Build history of the part. All positions in model axes, mm. Round coordinates to 2 decimals unless told otherwise and drop trailing zeros. Write each loop counter-clockwise with the first axis right and the second up, starting at its lowest first coordinate (ties: lowest second). Pieces come first, ordered by that corner, then holes. Notation, with made-up numbers: M -11.75,-36 L 14.25,-36 A11 ccw 14.25,-30 Z; hole C 70,-32.75 d5. An arc over 180 degrees is marked long. Write item = value, one per line.
Autodesk Inventor part; units mm, degrees
ref_plane "MP_XY" through (0, 0, 0) normal (0, 0, 1) x (1, 0, 0)
ref_plane "MP_YZ" through (0, 0, 0) normal (1, 0, 0) x (0, 1, 0)
ref_plane "MP_ZX" through (0, 0, 0) normal (0, 1, 0) x (0, 0, 1)
sketch "Sketch_12" plane through (0, 0, 0) normal (0, 0, 1) x (1, 0, 0)
  line L0 (-275, 538.5) -> (-275, 11.5)
  line L1 (-275, 11.5) -> (-273.5, 11.5)
  line L2 (-273.5, 11.5) -> (-263.9737, -5)
  line L3 (-263.9737, -5) -> (-255.5, -5)
  line L4 (-255.5, -5) -> (-255.5, 0)
  arc A0 (-244.5, 0) -> (-255.5, 0) centre (-250, 0) ccw
  line L5 (-244.5, 0) -> (-244.5, -12.5)
  line L6 (-244.5, -12.5) -> (244.5, -12.5)
  line L7 (244.5, -12.5) -> (244.5, 0)
  arc A1 (255.5, 0) -> (244.5, 0) centre (250, 0) ccw
  line L8 (255.5, 0) -> (255.5, -5)
  line L9 (255.5, -5) -> (263.9737, -5)
  line L10 (263.9737, -5) -> (273.5, 11.5)
  line L11 (273.5, 11.5) -> (275, 11.5)
  line L12 (275, 11.5) -> (275, 538.5)
  line L13 (275, 538.5) -> (273.5, 538.5)
  line L14 (273.5, 538.5) -> (263.9737, 555)
  line L15 (263.9737, 555) -> (255.5, 555)
  line L16 (255.5, 555) -> (255.5, 550)
  arc A2 (244.5, 550) -> (255.5, 550) centre (250, 550) ccw
  line L17 (244.5, 550) -> (244.5, 562.5)
  line L18 (244.5, 562.5) -> (-244.5, 562.5)
  line L19 (-244.5, 562.5) -> (-244.5, 550)
  arc A3 (-255.5, 550) -> (-244.5, 550) centre (-250, 550) ccw
  line L20 (-255.5, 550) -> (-255.5, 555)
  line L21 (-255.5, 555) -> (-263.9737, 555)
  line L22 (-263.9737, 555) -> (-273.5, 538.5)
  line L23 (-273.5, 538.5) -> (-275, 538.5)
  arc A4 (216.8088, 4.2) -> (216.8088, -4.2) centre (210, 0) ccw
  line L24 (216.8088, -4.2) -> (229, -4.2)
  line L25 (229, -4.2) -> (229, 4.2)
  line L26 (229, 4.2) -> (216.8088, 4.2)
  arc A5 (216.8088, 554.2) -> (216.8088, 545.8) centre (210, 550) ccw
  line L27 (216.8088, 545.8) -> (229, 545.8)
  line L28 (229, 545.8) -> (229, 554.2)
  line L29 (229, 554.2) -> (216.8088, 554.2)
  line L30 (-229, 4.2) -> (-229, -4.2)
  line L31 (-229, -4.2) -> (-216.8088, -4.2)
  arc A6 (-216.8088, -4.2) -> (-216.8088, 4.2) centre (-210, 0) ccw
  line L32 (-216.8088, 4.2) -> (-229, 4.2)
  line L33 (-229, 554.2) -> (-229, 545.8)
  line L34 (-229, 545.8) -> (-216.8088, 545.8)
  arc A7 (-216.8088, 545.8) -> (-216.8088, 554.2) centre (-210, 550) ccw
  line L35 (-216.8088, 554.2) -> (-229, 554.2)
extrude "Extrusion1" add sketch "Sketch_12" against normal blind 2.5
ref_plane "MP_XY" through (0, 0, 0) normal (0, 0, 1) x (1, 0, 0)
ref_plane "MP_YZ" through (0, 0, 0) normal (1, 0, 0) x (0, 1, 0)
ref_plane "MP_ZX" through (0, 0, 0) normal (0, 1, 0) x (0, 0, 1)
ref_plane "to_EB_XY" through (224.8, 0, -2.5) normal (0, 0, 1) x (1, 0, 0)
ref_plane "to_EB_YZ" through (224.8, 0, -2.5) normal (1, 0, 0) x (0, 1, 0)
ref_plane "to_EB_ZX" through (224.8, 0, -2.5) normal (0, 1, 0) x (0, 0, 1)
properties part number "166X_02_00_P6_(2)"
1. Band-saw the part on A-A (x = -210). List the corners of the cut face in (y, z).
Responses:
outline = M -12.5,-2.5 L -8,-2.5 L -8,0 L -12.5,0 Z; M 8,-2.5 L 542,-2.5 L 542,0 L 8,0 Z; M 558,-2.5 L 562.5,-2.5 L 562.5,0 L 558,0 Z
2. Mould opens along X. For faces 1 (the face through (-4, 279, 0)), 2 (the face through (-202, 550, -1)), 3 (the face through (202, 550, -1)) say: pulls with the +X half, pulls with the -X half, needs draft (parallel to the pull), parting line crosses it, or undercut.
Responses:
face_1 = needs draft
face_2 = undercut
face_3 = undercut
3. Probe probe 1 along Y at (x, z) = (-210, -1.4); probe 2 along Y at (x, z) = (-214.5, -0.8); probe 3 along X at (y, z) = (0, -1.6). List the from-to ranges inside material, lowest first.
Responses:
probe_1 = -12.5 to -8, 8 to 542, 558 to 562.5
probe_2 = -12.5 to -6.61, 6.61 to 543.39, 556.61 to 562.5
probe_3 = -266.86 to -255.5, -244.5 to -229, -202 to 202, 229 to 244.5, 255.5 to 266.86
4. Flat gauge pins, fed straight in: pin 1 (1.2 mm diameter, centred on x = -274, z = -1.5, fed in from -Y); pin 2 (1.2 mm diameter, centred on x = 258.5, z = -1.5, fed in from +Y); pin 3 (1.5 mm diameter, centred on x = -139, y = 357.5, fed in from +Z); pin 4 (1.2 mm diameter, centred on y = -2.5, z = -0.5, fed in from +X). Where does each tip first touch, or does it go through?
Responses:
pin_1 = 11.33
pin_2 = 555
pin_3 = 0
pin_4 = 265.76
